For this review, take the finished solid that the model builds, in its own axes (mm). A direction names the side the tool comes from. Round coordinates to 2 decimals unless told otherwise and drop trailing zeros. Write each loop counter-clockwise with the first axis right and the second up, starting at its lowest first coordinate (ties: lowest second). Pieces come first, ordered by that corner, then holes.
from build123d import *
from build123d.topology import SkipClean

# Parameters (mm, degrees)
SKETCH_1_W                = 85
SKETCH_1_H                = 30
EXTRUDE_1_DEPTH           = 11
SKETCH_2_W                = 27.5
SKETCH_2_H                = 5
CUT_EXTRUDE_3_DEPTH       = 3
CUT_EXTRUDE_5_DEPTH       = 33
SKETCH_8_R                = 15
SKETCH_8_R_2              = 8
EXTRUDE_6_DEPTH           = 20
SKETCH_9_W                = 4
SKETCH_9_H                = 21.735243828
CUT_EXTRUDE_6_DEPTH       = 20
SKETCH_10_R               = 4
EXTRUDE_7_DEPTH           = 21
SKETCH_11_R               = 6.5
CUT_EXTRUDE_9_DEPTH       = 40.5
SKETCH_13_R               = 6.5
EXTRUDE_8_DEPTH           = 18
SKETCH_14_R               = 4
CUT_EXTRUDE_10_DEPTH      = 18
SKETCH_15_R               = 8
CUT_EXTRUDE_11_DEPTH      = 18
CUT_EXTRUDE_12_DEPTH      = 18
CUT_EXTRUDE_13_DEPTH      = 58.984911924
CUT_EXTRUDE_13_DEPTH_BACK = 58.984911924
SKETCH_19_W               = 30
SKETCH_19_H               = 3


with BuildPart() as part:
    # Sketch 1 → Extrude 1 (new body)
    with BuildSketch(Plane.XY):
        Rectangle(SKETCH_1_W, SKETCH_1_H)
    extrude(amount=EXTRUDE_1_DEPTH)

    # Sketch 2 → Cut-Extrude 3 (cut)
    with BuildSketch(Plane.XY):
        with Locations((-28.75, 12.5)):
            Rectangle(SKETCH_2_W, SKETCH_2_H)
        with Locations((28.75, 12.5)):
            Rectangle(SKETCH_2_W, SKETCH_2_H)
        with Locations((28.75, -12.5)):
            Rectangle(SKETCH_2_W, SKETCH_2_H)
        with Locations((-28.75, -12.5)):
            Rectangle(SKETCH_2_W, SKETCH_2_H)
    extrude(amount=CUT_EXTRUDE_3_DEPTH, mode=Mode.SUBTRACT)

    # Sketch 6 → Cut-Extrude 5 (cut)
    with BuildSketch(Plane.XY):
        with BuildLine():
            Line((-35, 4), (-30, 4))
            ThreePointArc((-30, 4), (-26, 0), (-30, -4))
            Line((-30, -4), (-35, -4))
            ThreePointArc((-35, -4), (-39, 0), (-35, 4))
        make_face()
        with BuildLine():
            Line((35, 4), (30, 4))
            ThreePointArc((30, 4), (26, 0), (30, -4))
            Line((30, -4), (35, -4))
            ThreePointArc((35, -4), (39, 0), (35, 4))
        make_face()
    extrude(amount=CUT_EXTRUDE_5_DEPTH, mode=Mode.SUBTRACT)

    # Sketch 8 → Extrude 6 (add, symmetric)
    with BuildSketch(Plane(origin=(0, 0, 0), x_dir=(1, 0, 0), z_dir=(0, 1, 0))):
        with Locations(Location((0, 14, 0), (0, 0, 270))):
            Circle(SKETCH_8_R)
        with Locations(Location((0, 14, 0), (0, 0, 270))):
            Circle(SKETCH_8_R_2, mode=Mode.SUBTRACT)
    extrude(amount=EXTRUDE_6_DEPTH, both=True)

    # Sketch 9 → Cut-Extrude 6 (cut, symmetric)
    with BuildSketch(Plane(origin=(0, 0, 0), x_dir=(1, 0, 0), z_dir=(0, 1, 0))):
        with Locations((0, 31.336277545)):
            Rectangle(SKETCH_9_W, SKETCH_9_H)
    extrude(amount=CUT_EXTRUDE_6_DEPTH, both=True, mode=Mode.SUBTRACT)

    # Sketch 10 → Extrude 7 (add, symmetric)
    with BuildSketch(Plane(origin=(0, 0, 0), x_dir=(0, 0, -1), z_dir=(1, 0, 0))):
        with BuildLine():
            Line((0, 10), (0, -10))
            Line((0, -10), (24, -10))
            ThreePointArc((24, -10), (34, 0), (24, 10))
            Line((24, 10), (0, 10))
        make_face()
        with Locations(Location((24, 0, 0), (0, 0, 180))):
            Circle(SKETCH_10_R, mode=Mode.SUBTRACT)
    extrude(amount=EXTRUDE_7_DEPTH, both=True)

    # Sketch 11 → Cut-Extrude 9 (cut, symmetric)
    with BuildSketch(Plane(origin=(0, 0, 0), x_dir=(0, 0, -1), z_dir=(1, 0, 0))):
        with Locations((24, 0)):
            Circle(SKETCH_11_R)
    extrude(amount=CUT_EXTRUDE_9_DEPTH, both=True, mode=Mode.SUBTRACT)

    # Sketch 13 → Extrude 8 (add, symmetric)
    with BuildSketch(Plane(origin=(0, 0, 0), x_dir=(0, 0, -1), z_dir=(1, 0, 0))):
        with Locations((24, 0)):
            Circle(SKETCH_13_R)
    extrude(amount=EXTRUDE_8_DEPTH, both=True)

    # Sketch 14 → Cut-Extrude 10 (cut, symmetric)
    with BuildSketch(Plane(origin=(0, 0, 0), x_dir=(0, 0, -1), z_dir=(1, 0, 0))):
        with Locations((24, 0)):
            Circle(SKETCH_14_R)
    extrude(amount=CUT_EXTRUDE_10_DEPTH, both=True, mode=Mode.SUBTRACT)

    # Sketch 15 → Cut-Extrude 11 (cut, symmetric)
    with BuildSketch(Plane(origin=(0, 0, 0), x_dir=(1, 0, 0), z_dir=(0, 1, 0))):
        with Locations(Location((0, 14, 0), (0, 0, 104.477512186))):
            Circle(SKETCH_15_R)
    extrude(amount=CUT_EXTRUDE_11_DEPTH, both=True, mode=Mode.SUBTRACT)

    # Sketch 16 → Cut-Extrude 12 (cut, symmetric)
    with SkipClean():  # the faces are left unmerged after this step: merging them gives an invalid solid
        with BuildSketch(Plane(origin=(0, 0, 0), x_dir=(1, 0, 0), z_dir=(0, 1, 0))):
            with BuildLine():
                Line((-2, 34), (2, 34))
                Line((2, 34), (2, 21.745966692))
                ThreePointArc((2, 21.745966692), (0, 22), (-2, 21.745966692))
                Line((-2, 21.745966692), (-2, 34))
            make_face()
        extrude(amount=CUT_EXTRUDE_12_DEPTH, both=True, mode=Mode.SUBTRACT)
    add(part.part.scale(1), mode=Mode.REPLACE)  # the faces are merged on a copy

    # Sketch 19 → Cut-Extrude 13 (cut, two sides: drawn at the far end of the back side and taken through both)
    with BuildSketch(Plane(origin=(0, 0, 0), x_dir=(1, 0, 0), z_dir=(0, 1, 0)).offset(-CUT_EXTRUDE_13_DEPTH_BACK)):
        with Locations((0, -9.5)):
            Rectangle(SKETCH_19_W, SKETCH_19_H)
    extrude(amount=CUT_EXTRUDE_13_DEPTH + CUT_EXTRUDE_13_DEPTH_BACK, mode=Mode.SUBTRACT)


solid = part.part
(1) We need section D-D, the plane y = 0. State how many separate pieces and enclosed holes the cut face has, and give its area (3 significant figures).
Geometry check:
separate pieces: 5
enclosed holes: 0
area: 1,410 mm2
(2) For pin 1 Ø2.5 at (x, z) = (-32.5, 5) entering from -Y; pin 2 Ø3 at (x, z) = (19, -17) entering from +Y; pin 3 Ø10.5 at (y, z) = (-0.5, -24) entering from +X, all flat-tipped, find the tip position at first contact; note any pin that passes through.
Geometry check:
pin 1: stops at y = -15
pin 2: stops at y = 10
pin 3: stops at x = 18
(3) For line 1 along X through (y, z) = (0, 1.5); line 2 along X through (y, z) = (0.5, -13.5); line 3 along X through (y, z) = (13.5, -13.5), list the stretches that pass through material, from the lowest coordinate up.
Geometry check:
line 1: x = -42.5 to -39, -26 to 26, 39 to 42.5
line 2: x = -21 to -7.98, 7.98 to 21
line 3: x = -14.99 to -7.98, 7.98 to 14.99
(4) We need section A-A, the plane z = -13. Give the boundary of the cut face in (x, y).
Geometry check:
outline: (-21, -10) - (-14.97, -10) - (-14.97, -20) - (-7.94, -20) - (-7.94, 20) - (-14.97, 20) - (-14.97, 10) - (-21, 10) - close; (7.94, -20) - (14.97, -20) - (14.97, -10) - (21, -10) - (21, 10) - (14.97, 10) - (14.97, 20) - (7.94, 20) - close
(5) Mouldability with a two-part tool opening along X and no side actions: class faces 5 (the face through (-15, 0, 10)), 6 (the face through (-18, 3, -27)), 7 (the face through (-1, -15, 7)) as pulls with the +X half, pulls with the -X half, needs draft (parallel to the pull), parting line crosses it, or undercut.
Geometry check:
face 5: undercut
face 6: pulls with the -X half
face 7: needs draft
(6) For faces 1 (the face through (-29, 13, 3)), 2 (the face through (-11, 0, -34)), 3 (the face through (12, 0, -34)), 4 (the face through (-26, 0, 5)), list the 3-axis set-ups (+Z, -Z, +X, -X, +Y, -Y) from which the entire face can be reached by the end or side of a thin tool; tool diameter is ignored.
Geometry check:
face 1: -Z, -X, +Y
face 2: -Z, -X
face 3: -Z, +X
face 4: +Z, -Z
(7) We need section C-C, the plane z = -5. Give the boundary of the cut face in (x, y).
Geometry check:
outline: (-21, -10) - (-12, -10) - (-12, -20) - (12, -20) - (12, -10) - (21, -10) - (21, 10) - (12, 10) - (12, 20) - (-12, 20) - (-12, 10) - (-21, 10) - close
(8) We need section B-B, the plane x = 0. Give the boundary of the cut face in (y, z), and give its area (3 significant figures).
Geometry check:
outline: (-20, -6) - (20, -6) - (20, 1) - (15, 1) - (15, 8) - (-15, 8) - (-15, 1) - (-20, 1) - close
area: 490 mm2
